Can you work these out from the drawing? Everything is in mm from the part's minimum corner. Coordinates: 2 decimals unless noted, no trailing zeros. Write each loop counter-clockwise with the first axis right and the second up, starting at its lowest first coordinate (ties: lowest second). Pieces come first, ordered by that corner, then holes. Notation, with made-up numbers: (83, 43.25) -> (140, 43.25) arc R8 cw to (140, 48.25) -> close; hole circle Ø7 at (-7.5, 17.25). An arc over 180 degrees is marked (long way). Use a Markdown table: item, result. Add a question column.
Item 1: Will these pins go through, and if not, where does the flat tip stop? pin 1 Ø1.5 at (y, z) = (17.5, 26) entering from -X; pin 2 Ø1.5 at (x, z) = (77.5, 35) entering from -Y; pin 3 Ø9 at (x, z) = (363.5, 36.5) entering from -Y; pin 4 Ø0.9 at (y, z) = (18, 27.5) entering from +X.
Item 2: Imagine slicing it at A-A, the plane z = 16.5. Write out the boundary of the cut face in (x, y).
Item 3: If I drill on line 1 along X through (y, z) = (2.5, 3), over which ranges is the centre line in solid material (lowest first)? Write a range as from..to.
Item 4: Imagine slicing it at B-B, the plane y = 4.75. Write out the boundary of the cut face in (x, z).
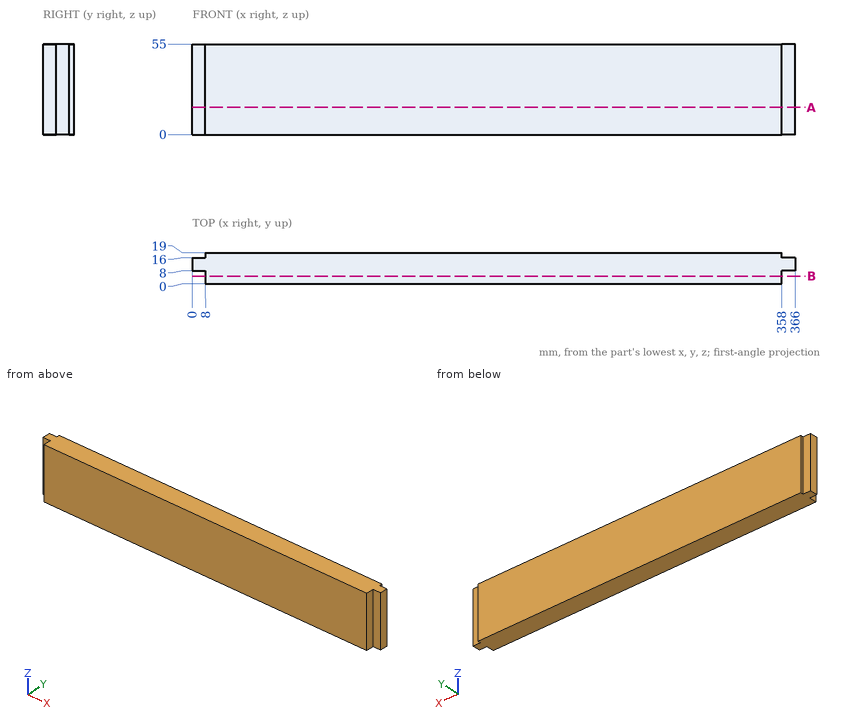
Ans:
| question | item | result |
|---|---|---|
| 1 | pin 1 | stops at x = 8 |
| 1 | pin 2 | stops at y = 0 |
| 1 | pin 3 | stops at y = 8 |
| 1 | pin 4 | stops at x = 358 |
| 2 | outline | (0, 8) -> (8, 8) -> (8, 0) -> (358, 0) -> (358, 8) -> (366, 8) -> (366, 16) -> (358, 16) -> (358, 19) -> (8, 19) -> (8, 16) -> (0, 16) -> close |
| 3 | line 1 | x = 8..358 |
| 4 | outline | (8, 0) -> (358, 0) -> (358, 55) -> (8, 55) -> close |
